Design review of the part built by this model. Coordinates are the model's own, in mm. A direction names the side the tool comes from. Give positions to 0.01 mm unless a question says otherwise; leave off trailing zeros. Put each result on its own line as item: value. Start each with the question number.
from build123d import *

# Parameters (mm, degrees)
SHELL_1_T                = -3
CUT_EXTRUDE_START        = 55
SKETCH_4_W               = 17
SKETCH_4_H               = 30
CUT_EXTRUDE_1_DEPTH      = 36.807488848
CUT_EXTRUDE_START_2      = -55
SKETCH_4_2_W             = 17
SKETCH_4_2_H             = 30
CUT_EXTRUDE_2_DEPTH      = 36.807488848
EXTRUDE_START            = 55
SKETCH_4_3_W             = 17
SKETCH_4_3_H             = 30
EXTRUDE_1_DEPTH          = 2
EXTRUDE_START_2          = -55
SKETCH_4_4_W             = 17
SKETCH_4_4_H             = 30
EXTRUDE_2_DEPTH          = 2
SKETCH_5_R               = 1.6
EXTRUDE_3_DEPTH          = 110
CUT_EXTRUDE_3_DEPTH      = 93.390042924
CUT_EXTRUDE_3_DEPTH_BACK = 93.390042924
SKETCH_5_3_R             = 0.6
CUT_EXTRUDE_4_DEPTH      = 15
CUT_EXTRUDE_4_DEPTH_BACK = 15
SKETCH_5_4_R             = 1.6
SKETCH_5_4_R_2           = 0.6
CUT_EXTRUDE_START_3      = -43
SKETCH_5_5_R             = 1.6
SKETCH_5_5_R_2           = 0.6
CUT_EXTRUDE_5_DEPTH      = 50.390042924
CUT_EXTRUDE_START_4      = 43
SKETCH_5_6_R             = 1.6
SKETCH_5_6_R_2           = 0.6
CUT_EXTRUDE_6_DEPTH      = 50.390042924
CUT_EXTRUDE_8_DEPTH      = 137.787865114
EXTRUDE_4_DEPTH          = 2


with BuildPart() as part:
    # 草图1 → 放样1 section 0
    with BuildSketch(Plane(origin=(0, 0, 0), x_dir=(1, 0, 0), z_dir=(0, 1, 0))):
        with BuildLine():
            Line((-50, -30), (50, -30))
            Line((50, -30), (50, 30))
            Line((50, 30), (-50, 30))
            Line((-50, 30), (-50, -30))
        make_face()
    # 草图2 → 放样1 section 1
    with BuildSketch(Plane(origin=(0, 50, 0), x_dir=(1, 0, 0), z_dir=(0, 1, 0))):
        with BuildLine():
            Line((-65, -39), (65, -39))
            Line((65, -39), (65, 39))
            Line((65, 39), (-65, 39))
            Line((-65, 39), (-65, -39))
        make_face()
    loft()

    # 抽壳1
    shell_1_openings = [part.faces().sort_by_distance(p)[0] for p in [
        (0, 50, 0),
    ]]
    offset(amount=SHELL_1_T, openings=shell_1_openings, kind=Kind.INTERSECTION)

    # 草图4 → 切除-拉伸1 (cut, through all)
    with BuildSketch(Plane(origin=(0, 0, 0), x_dir=(0, 0, -1), z_dir=(1, 0, 0)).offset(CUT_EXTRUDE_START)):
        with Locations((-30.5, 35)):
            Rectangle(SKETCH_4_W, SKETCH_4_H)
    extrude(amount=CUT_EXTRUDE_1_DEPTH, mode=Mode.SUBTRACT)

    # 草图4<2> → 切除-拉伸2 (cut, through all)
    with BuildSketch(Plane(origin=(0, 0, 0), x_dir=(0, 0, -1), z_dir=(1, 0, 0)).offset(CUT_EXTRUDE_START_2)):
        with Locations((-30.5, 35)):
            Rectangle(SKETCH_4_2_W, SKETCH_4_2_H)
    extrude(amount=-CUT_EXTRUDE_2_DEPTH, mode=Mode.SUBTRACT)

    # 草图4<3> → 凸台-拉伸1 (add)
    with BuildSketch(Plane(origin=(0, 0, 0), x_dir=(0, 0, -1), z_dir=(1, 0, 0)).offset(EXTRUDE_START)):
        with Locations((-30.5, 35)):
            Rectangle(SKETCH_4_3_W, SKETCH_4_3_H)
    extrude(amount=-EXTRUDE_1_DEPTH)

    # 草图4<4> → 凸台-拉伸2 (add)
    with BuildSketch(Plane(origin=(0, 0, 0), x_dir=(0, 0, -1), z_dir=(1, 0, 0)).offset(EXTRUDE_START_2)):
        with Locations((-30.5, 35)):
            Rectangle(SKETCH_4_4_W, SKETCH_4_4_H)
    extrude(amount=EXTRUDE_2_DEPTH)

    # 草图5 → 凸台-拉伸3 (add)
    with BuildSketch(Plane(origin=(0, 0, 0), x_dir=(0, 0, -1), z_dir=(1, 0, 0)).offset(EXTRUDE_START)):
        with Locations((-39, 50)):
            Circle(SKETCH_5_R)
    extrude(amount=-EXTRUDE_3_DEPTH)

    # 草图5<3> → 切除-拉伸3 (cut, two sides: drawn at the far end of the back side and taken through both)
    with BuildSketch(Plane(origin=(0, 0, 0), x_dir=(0, 0, -1), z_dir=(1, 0, 0)).offset(-CUT_EXTRUDE_3_DEPTH_BACK)):
        with Locations((-39, 50)):
            Circle(SKETCH_5_3_R)
    extrude(amount=CUT_EXTRUDE_3_DEPTH + CUT_EXTRUDE_3_DEPTH_BACK, mode=Mode.SUBTRACT)

    # 草图5<4> → 切除-拉伸4 (cut, two sides: drawn at the far end of the back side and taken through both)
    with BuildSketch(Plane(origin=(0, 0, 0), x_dir=(0, 0, -1), z_dir=(1, 0, 0)).offset(-CUT_EXTRUDE_4_DEPTH_BACK)):
        with Locations((-39, 50)):
            Circle(SKETCH_5_4_R)
        with Locations((-39, 50)):
            Circle(SKETCH_5_4_R_2, mode=Mode.SUBTRACT)
    extrude(amount=CUT_EXTRUDE_4_DEPTH + CUT_EXTRUDE_4_DEPTH_BACK, mode=Mode.SUBTRACT)

    # 草图5<5> → 切除-拉伸5 (cut, through all)
    with BuildSketch(Plane(origin=(0, 0, 0), x_dir=(0, 0, -1), z_dir=(1, 0, 0)).offset(CUT_EXTRUDE_START_3)):
        with Locations((-39, 50)):
            Circle(SKETCH_5_5_R)
        with Locations((-39, 50)):
            Circle(SKETCH_5_5_R_2, mode=Mode.SUBTRACT)
    extrude(amount=-CUT_EXTRUDE_5_DEPTH, mode=Mode.SUBTRACT)

    # 草图5<6> → 切除-拉伸6 (cut, through all)
    with BuildSketch(Plane(origin=(0, 0, 0), x_dir=(0, 0, -1), z_dir=(1, 0, 0)).offset(CUT_EXTRUDE_START_4)):
        with Locations((-39, 50)):
            Circle(SKETCH_5_6_R)
        with Locations((-39, 50)):
            Circle(SKETCH_5_6_R_2, mode=Mode.SUBTRACT)
    extrude(amount=CUT_EXTRUDE_6_DEPTH, mode=Mode.SUBTRACT)

    # 草图6 → 切除-拉伸8 (cut, through all)
    with BuildSketch(Plane(origin=(55, 0, 0), x_dir=(0, 0, -1), z_dir=(1, 0, 0))):
        Polygon((-39, 20), (-33.6, 20), (-38.1, 45), (-39, 45), align=None)
    extrude(amount=-CUT_EXTRUDE_8_DEPTH, mode=Mode.SUBTRACT)

    # 草图7 → 凸台-拉伸4 (add)
    with BuildSketch(Plane(origin=(0, 0, 22), x_dir=(-1, 0, 0), z_dir=(0, 0, -1))):
        Polygon((-65, 50), (-56, 20), (-53, 20), (-53, 50), align=None)
        Polygon((65, 50), (56, 20), (53, 20), (53, 50), align=None)
    extrude(amount=EXTRUDE_4_DEPTH)


solid = part.part
1. To check wall thickness, follow probe 1 along Y at (x, z) = (21.5, 39); probe 2 along Y at (x, z) = (-40, -26.5); probe 3 along X at (y, z) = (6, -5.5). State the ranges of each line that lie inside material, in increasing order.
2. Insertion check: pin 1 (4 mm diameter, centred on x = 49.5, y = 38.5, fed in from -Z); pin 2 (1.6 mm diameter, centred on x = 54, y = 46.5, fed in from +Z); pin 3 (5 mm diameter, centred on x = 58, y = 35, fed in from +Z). Each pin has a flat end and moves straight along its axis. Give the tip position at first contact, or say it passes through.
3. Machinability: for faces 1 (the flat face through (1, 50, -37)), 2 (the flat face through (-43, 50, 38)), 3 (the flat face through (-0.74, 26.83, 31.78)), 4 (the flat face through (15, 50, 38)), 5 (the flat face through (43, 50, 38)), which of the approach directions +Z, -Z, +X, -X, +Y, -Y give a long, thin tool a straight path to every point of the face, cutting with its end or side? Answer none if there is none.
Returned:
1. probe 1: y = 48.4 to 49.4, 50.6 to 51.6
1. probe 2: y = 0 to 3
1. probe 3: x = -51.8 to -48.67, 48.67 to 51.8
2. pin 1: stops at z = -37.29
2. pin 2: stops at z = 39
2. pin 3: stops at z = 22
3. face 1: -Z, +X, -X, +Y
3. face 2: +Z, -X, +Y
3. face 3: +Y
3. face 4: +Z, +Y
3. face 5: +Z, +X, +Y
